Could you check a few things on this drawing? It's one solid part, dimensions in mm from its lowest x, y, z. A direction names the side the tool comes from. Round coordinates to 2 decimals unless told otherwise and drop trailing zeros. Loops run counter-clockwise (first coordinate to the right, second up) from the corner with the lowest first, then second, coordinate; pieces in that order, holes last. Notation, with made-up numbers: (72, 7) -> (124, 7) arc R20 cw to (124, 39) -> close; hole circle Ø11 at (-5, 56.5). An arc over 180 degrees is marked (long way). Put each result on its own line as item: value. Start each with the question number.
1. Which directions (+Z, -Z, +X, -X, +Y, -Y) give clear straight access to the entire face, cutting with the end or side of a thin tool? Please do the marked faces 3 and 4.
2. Imagine slicing it at C-C, the plane y = 3.25. Please give me the cut outline in (x, z), and give its area (3 significant figures).
3. Imagine slicing it at B-B, the plane x = 40. Please give me the cut outline in (y, z).
4. Imagine slicing it at A-A, the plane z = 40. Please give me the cut outline in (x, y), and give its area (3 significant figures).
5. If we mould it in two halves opening along X, with no side actions, what happens to the marked faces 1 and 2? For each: pulls with the +X half, pulls with the -X half, needs draft (parallel to the pull), parting line crosses it, or undercut.
6. I'm going to push flat-ended pins straight in: P1, Ø4, axis at x = 55, y = 7, coming from the -Z side; P2, Ø3, axis at y = 7, z = 43, coming from the +X side; P3, Ø5, axis at x = 43.5, y = 2, coming from the -Z side. Where does each tip first touch, or does it pass through?
7. I need wall thicknesses on line 1 (X direction, y = 7, z = 40); line 2 (X direction, y = 4.25, z = 40); line 3 (Y direction, x = 54, z = 3.5). Which ranges of each line are inside material? Lowest first, please. Write a range as [from, to].
8. Imagine slicing it at D-D, the plane x = 72. Please give me the cut outline in (y, z), and give its area (3 significant figures).
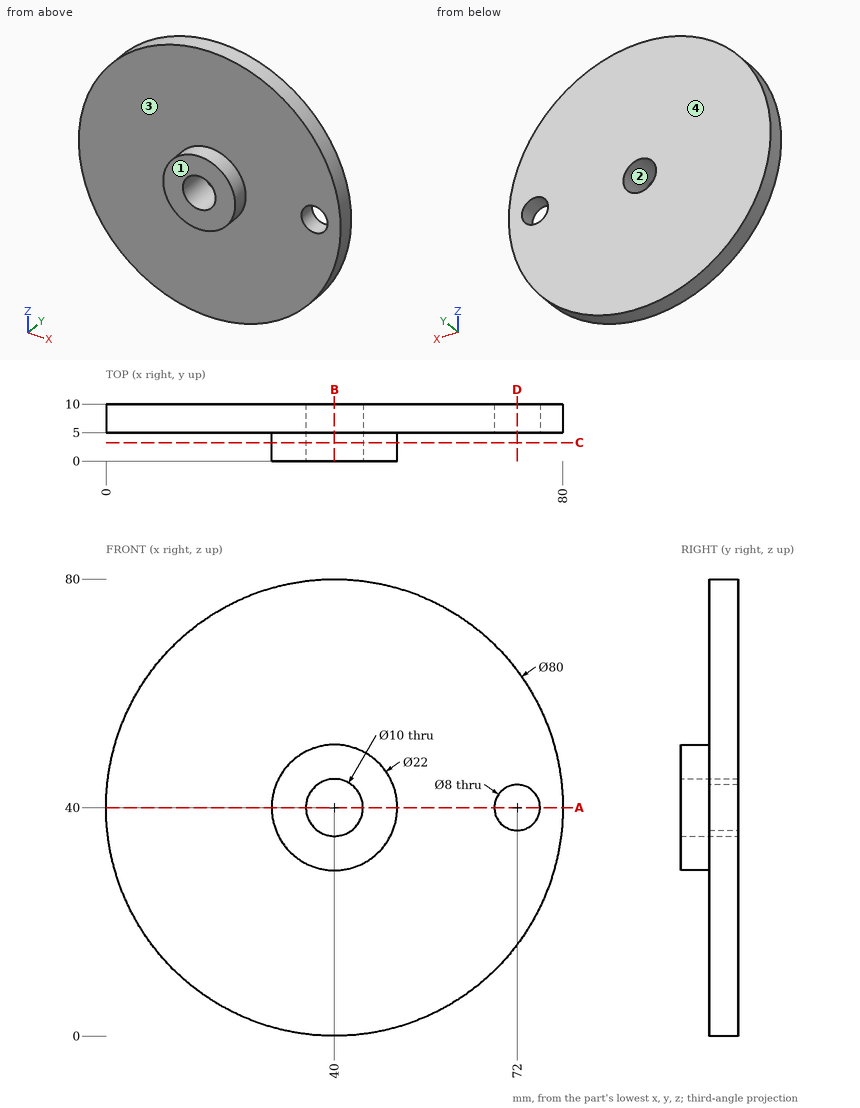
Entries:
1. face 3: -Y
1. face 4: +Z, -Z, +X, -X, +Y
2. outline: circle Ø22 at (40, 40); hole circle Ø10 at (40, 40)
2. area: 302 mm^2
3. outline: (0, 29) -> (5, 29) -> (5, 0) -> (10, 0) -> (10, 35) -> (0, 35) -> close; (0, 45) -> (10, 45) -> (10, 80) -> (5, 80) -> (5, 51) -> (0, 51) -> close
4. outline: (0, 5) -> (29, 5) -> (29, 0) -> (35, 0) -> (35, 10) -> (0, 10) -> close; (45, 0) -> (51, 0) -> (51, 5) -> (68, 5) -> (68, 10) -> (45, 10) -> close; (76, 5) -> (80, 5) -> (80, 10) -> (76, 10) -> close
4. area: 370 mm^2
5. face 1: needs draft
5. face 2: undercut
6. P1: z = 2.17
6. P2: x = 79.97
6. P3: z = 29.05
7. line 1: [0, 35], [45, 68], [76, 80]
7. line 2: [29, 35], [45, 51]
7. line 3: [5, 10]
8. outline: (5, 16) -> (10, 16) -> (10, 36) -> (5, 36) -> close; (5, 44) -> (10, 44) -> (10, 64) -> (5, 64) -> close
8. area: 200 mm^2
